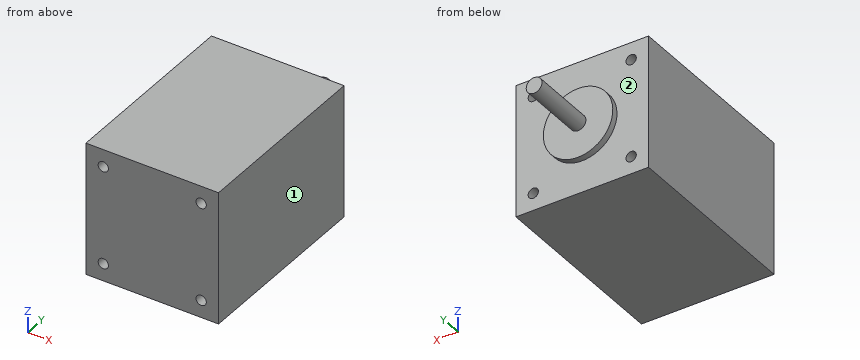
from build123d import *

# Parameters (mm, degrees)
SKETCH_1_W          = 42
SKETCH_1_H          = 42
EXTRUDE_1_DEPTH     = 60
SKETCH_2_R          = 11
EXTRUDE_2_DEPTH     = 2
SKETCH_3_R          = 2.5
EXTRUDE_3_DEPTH     = 21
SKETCH_4_R          = 1.625
CUT_EXTRUDE_1_DEPTH = 85.427483677


with BuildPart() as part:
    # 草图1 → 凸台-拉伸1 (new body)
    with BuildSketch(Plane(origin=(0, 0, 0), x_dir=(1, 0, 0), z_dir=(0, 1, 0))):
        with Locations((21, 21)):
            Rectangle(SKETCH_1_W, SKETCH_1_H)
    extrude(amount=EXTRUDE_1_DEPTH)

    # 草图2 → 凸台-拉伸2 (add)
    with BuildSketch(Plane(origin=(0, 60, 0), x_dir=(1, 0, 0), z_dir=(0, 1, 0))):
        with Locations(Location((21, 21, 0), (0, 0, 270))):
            Circle(SKETCH_2_R)
    extrude(amount=EXTRUDE_2_DEPTH)

    # 草图3 → 凸台-拉伸3 (add)
    with BuildSketch(Plane(origin=(0, 62, 0), x_dir=(1, 0, 0), z_dir=(0, 1, 0))):
        with Locations(Location((21, 21, 0), (0, 0, 90))):
            Circle(SKETCH_3_R)
    extrude(amount=EXTRUDE_3_DEPTH)

    # 草图4 → 切除-拉伸1 (cut, through all)
    with BuildSketch(Plane(origin=(0, 60, 0), x_dir=(1, 0, 0), z_dir=(0, 1, 0))):
        with Locations(Location((5.5, 36.5, 0), (0, 0, 270))):
            Circle(SKETCH_4_R)
        with Locations(Location((36.5, 36.5, 0), (0, 0, 270))):
            Circle(SKETCH_4_R)
        with Locations(Location((36.5, 5.5, 0), (0, 0, 270))):
            Circle(SKETCH_4_R)
        with Locations(Location((5.5, 5.5, 0), (0, 0, 270))):
            Circle(SKETCH_4_R)
    extrude(amount=-CUT_EXTRUDE_1_DEPTH, mode=Mode.SUBTRACT)


solid = part.part
Input: part model. Units: mm. Frame: model coordinates. Face numbers are marked on the shaded views. A direction names the side the tool comes from. Coordinates: 2 decimals unless noted, no trailing zeros. Order: outer loops, then holes, each group sorted by start corner. A loop starts at its lowest first (then second) coordinate and runs counter-clockwise, first axis right, second up. Notation, with made-up numbers: M 50.5,17.25 L 64.5,17.25 A19 cw 64.5,27.25 Z; hole C 10.25,-31 d3. An arc over 180 degrees is marked long. One line per question, with ' | ' between items.
Item 1: Section C-C (z = -5.5). Output: boundary loops of the cut face in (x, y) (3 decimals).
Geometry results:
outline: M 0,0 L 3.875,0 L 3.875,60 L 0,60 Z; M 7.125,0 L 34.875,0 L 34.875,60 L 7.125,60 Z; M 38.125,0 L 42,0 L 42,60 L 38.125,60 Z
Item 2: Ray query, line 1 along X through (y, z) = (38.5, -36.5) (3 decimals); line 2 along X through (y, z) = (56, -35.5); line 3 along Z through (x, y) = (5, 23). Return the intervals inside material, ascending.
Geometry results:
line 1: x = 0 to 3.875, 7.125 to 34.875, 38.125 to 42 | line 2: x = 0 to 4.22, 6.78 to 35.22, 37.78 to 42 | line 3: z = -42 to -38.05, -34.95 to -7.05, -3.95 to 0
Item 3: Reachability of the marked faces 1 and 2 from +Z, -Z, +X, -X, +Y, -Y: full face, straight path, thin tool, end or side. Return the list, or none.
Geometry results:
face 1: +Z, -Z, +X, +Y, -Y | face 2: +Y
Item 4: Section D-D (z = -21). Output: boundary loops of the cut face in (x, y), then the cut area to 3 significant figures.
Geometry results:
outline: M 0,0 L 42,0 L 42,60 L 32,60 L 32,62 L 23.5,62 L 23.5,83 L 18.5,83 L 18.5,62 L 10,62 L 10,60 L 0,60 Z | area: 2,670 mm^2
Item 5: Section A-A (y = 27.5). Output: boundary loops of the cut face in (x, z) (3 decimals).
Geometry results:
outline: M 0,-42 L 42,-42 L 42,0 L 0,0 Z; hole C 5.5,-36.5 d3.25; hole C 5.5,-5.5 d3.25; hole C 36.5,-36.5 d3.25; hole C 36.5,-5.5 d3.25
Item 6: Pin query (flat end, axial travel): pin 1 (1 mm diameter, centred on x = 19.5, y = 65.5, fed in from -Z); pin 2 (4 mm diameter, centred on x = 36.5, z = -5.5, fed in from +Y); pin 3 (3 mm diameter, centred on x = 5.5, z = -36.5, fed in from +Y); pin 4 (6 mm diameter, centred on x = 28, z = -32.5, fed in from +Y). Return the tip coordinate at first contact, or that it passes through.
Geometry results:
pin 1: stops at z = -23.29 | pin 2: stops at y = 60 | pin 3: passes through | pin 4: stops at y = 62
Item 7: Section B-B (x = 36.5). Output: boundary loops of the cut face in (y, z) (3 decimals), then the cut area to 3 significant figures.
Geometry results:
outline: M 0,-42 L 60,-42 L 60,-38.125 L 0,-38.125 Z; M 0,-34.875 L 60,-34.875 L 60,-7.125 L 0,-7.125 Z; M 0,-3.875 L 60,-3.875 L 60,0 L 0,0 Z | area: 2,130 mm^2
